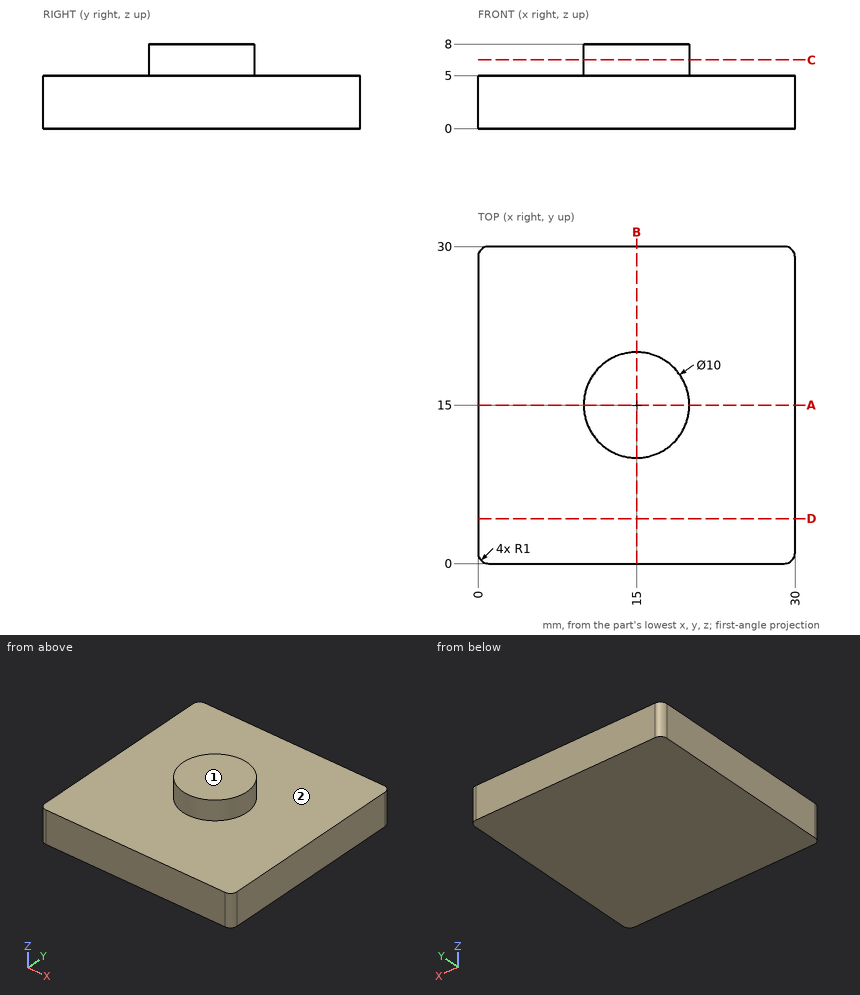
Geometry: see drawing. Coordinates: mm, zero at the bounding-box minimum. A direction names the side the tool comes from. Round coordinates to 2 decimals unless told otherwise and drop trailing zeros. Write each loop counter-clockwise with the first axis right and the second up, starting at its lowest first coordinate (ties: lowest second). Pieces come first, ordered by that corner, then holes. Notation, with made-up numbers: (64, 18.25) - (103, 18.25) arc R28 cw to (103, 41.25) - close; hole circle Ø11 at (-16.5, 23.25). An arc over 180 degrees is marked (long way). Use CSV: the item, a comma, the result in double quotes. Start each with the question number.
(1) Material intervals for probe 1 along Z at (x, y) = (11.25, 2); probe 2 along Y at (x, z) = (13.75, 5.5); probe 3 along Y at (x, z) = (16.75, 7.5), sorted ascending. Write a range as [from, to].
(2) Cut plane A-A, the plane y = 15. Return loops of the section in (x, z).
(3) Set-up query: the marked faces 1 and 2. Return all of +Z, -Z, +X, -X, +Y, -Y with unobstructed straight access to the full face (end or side cutting, diameter ignored); none if empty.
(4) Cut plane C-C, the plane z = 6.5. Return loops of the section in (x, y), and give its area (3 significant figures).
(5) First-contact query: pin 1 Ø12 at (x, y) = (4, 24) entering from +Z. Flat tip, straight axial feed; report the tip coordinate or a pass-through.
(6) Cut plane D-D, the plane y = 4.25. Return loops of the section in (x, z).
Geometry says:
1,probe 1,"[0, 5]"
1,probe 2,"[10.16, 19.84]"
1,probe 3,"[10.32, 19.68]"
2,outline,"(0, 0) - (30, 0) - (30, 5) - (20, 5) - (20, 8) - (10, 8) - (10, 5) - (0, 5) - close"
3,face 1,"+Z, +X, -X, +Y, -Y"
3,face 2,"+Z"
4,outline,"circle Ø10 at (15, 15)"
4,area,"78.5 mm²"
5,pin 1,"z = 5"
6,outline,"(0, 0) - (30, 0) - (30, 5) - (0, 5) - close"
